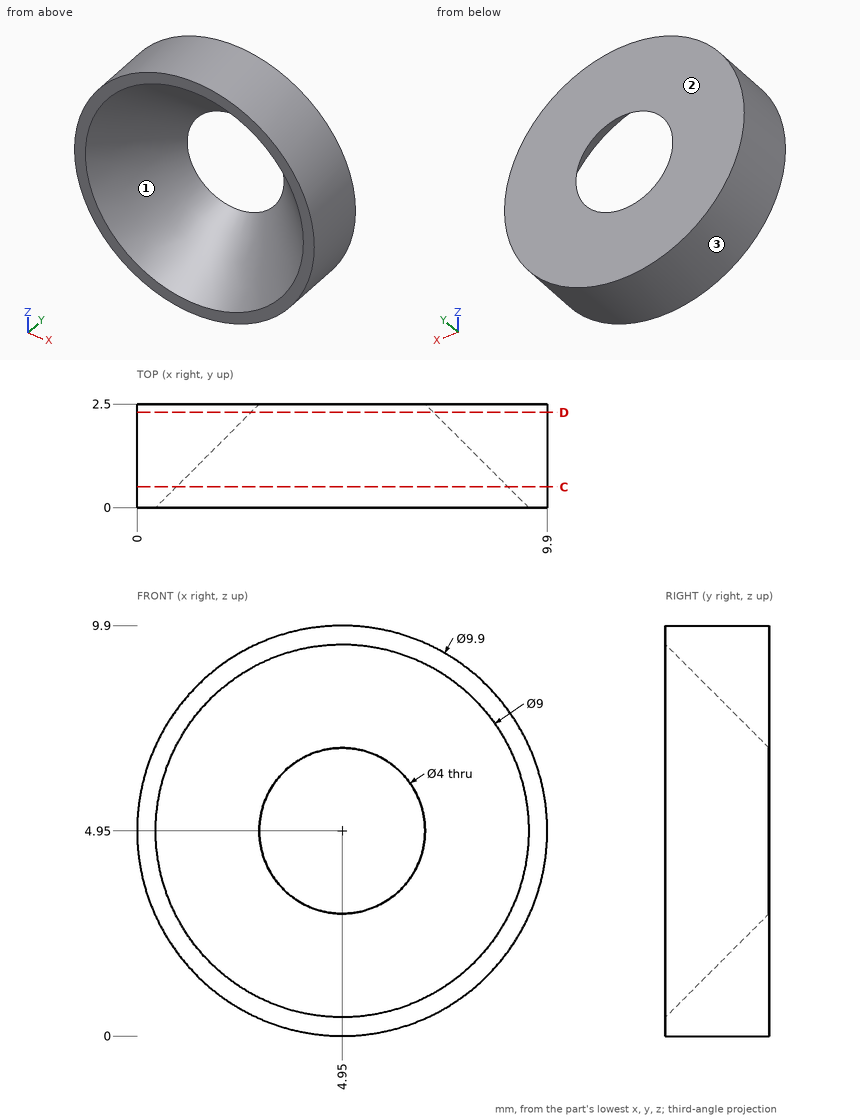
The figure shows three views and two pictorial views of one solid part (mm, origin at its lowest corner). Answer the questions. Give positions to 0.01 mm unless a question says otherwise; leave off trailing zeros. Write each loop counter-clockwise with the first axis right and the second up, starting at its lowest first coordinate (ties: lowest second). Pieces come first, ordered by that corner, then holes.
Q1. The part is cut by section C-C on y = 0.5. Give the vertices of the cut face in (x, z), and give its area (3 significant figures).
Answer:
outline: circle Ø9.9 at (4.95, 4.95); hole circle Ø8 at (4.95, 4.95)
area: 26.7 mm2
Q2. Straight lines are drawn through the part: L1, parallel to X at y = 0.9, z = 2 (1 decimal); L2, parallel to Z at x = 5, y = 1.55; L3, parallel to X at y = 0.7, z = 2 (3 decimals). For each, find the intervals that lie inside material, in ascending order.
Answer:
L1: x = 1 to 2.9, 7 to 8.9
L2: z = 0 to 2, 7.9 to 9.9
L3: x = 0.975 to 2.555, 7.345 to 8.925
Q3. The part is cut by section D-D on y = 2.3. Give the vertices of the cut face in (x, z), and give its area (3 significant figures).
Answer:
outline: circle Ø9.9 at (4.95, 4.95); hole circle Ø4.4 at (4.95, 4.95)
area: 61.8 mm2
Q4. For a pull along Z with two mould halves and no side action, classify the marked faces 1, 2 and 3 as released by +Z, released by -Z, zero draft, split by the parting line, or undercut.
Answer:
face 1: undercut
face 2: zero draft
face 3: split by the parting line
Q5. Given pin 1 (1 mm diameter, centred on x = 7.5, z = 4.5, fed in from -Y); pin 2 (2.5 mm diameter, centred on x = 4.95, z = 4.95, fed in from +Y), each flat-ended and moving along its own axis, determine where each tip first touches the part or whether it passes through.
Answer:
pin 1: stops at y = 1.41
pin 2: passes through
